Part print with two shaded views. Sizes in mm from the minimum x, y, z corner. Round coordinates to 2 decimals unless told otherwise and drop trailing zeros. Loops run counter-clockwise (first coordinate to the right, second up) from the corner with the lowest first, then second, coordinate; pieces in that order, holes last.
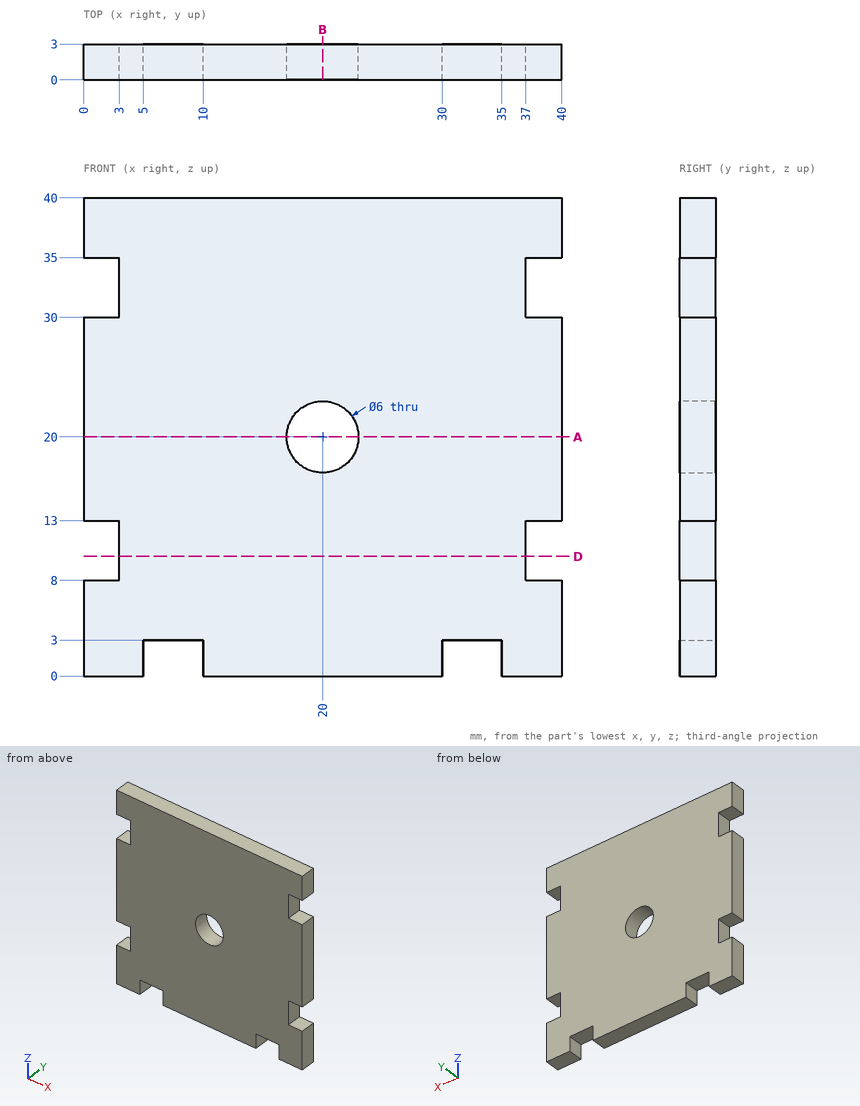
Item 1: Cut at D-D (z = 10). List the corners of the cut face in (x, y).
Verdict:
outline: (3, 0) - (37, 0) - (37, 3) - (3, 3) - close
Item 2: Cut at A-A (z = 20). List the corners of the cut face in (x, y), plus the area to 3 significant figures.
Verdict:
outline: (0, 0) - (17, 0) - (17, 3) - (0, 3) - close; (23, 0) - (40, 0) - (40, 3) - (23, 3) - close
area: 102 mm2
Item 3: Wall check: L1, parallel to X at y = 1.7, z = 20; L2, parallel to X at y = 2.2, z = 12.5; L3, parallel to Z at x = 32, y = 0.9. Give the ranges that are in metal, low to high.
Verdict:
L1: x = 0 to 17, 23 to 40
L2: x = 3 to 37
L3: z = 3 to 40
Item 4: Flat gauge pins, fed straight in: P1, Ø0.9, axis at x = 6.5, y = 2, coming from the -Z side; P2, Ø1, axis at y = 2.5, z = 15.5, coming from the -X side. Where does each tip first touch, or does it go through?
Verdict:
P1: stops at z = 3
P2: stops at x = 0
Item 5: Cut at B-B (x = 20). List the corners of the cut face in (y, z), plus the area to 3 significant figures.
Verdict:
outline: (0, 0) - (3, 0) - (3, 17) - (0, 17) - close; (0, 23) - (3, 23) - (3, 40) - (0, 40) - close
area: 102 mm2
